Can you work these out from the model? Positions are in its coordinate system, mm. Face numbers are marked on the shaded views. A direction names the side the tool comes from. Give positions to 0.01 mm unless a question says otherwise; leave off trailing zeros. Loops run counter-clockwise (first coordinate to the right, second up) from the corner with the lowest first, then second, coordinate; pieces in that order, holes last. Notation, with made-up numbers: M 74,40.5 L 117,40.5 A22 cw 117,75.5 Z; hole C 75.5,-28 d2. An arc over 180 degrees is marked long. Use CSV: the item, a comma, the result in double quotes.
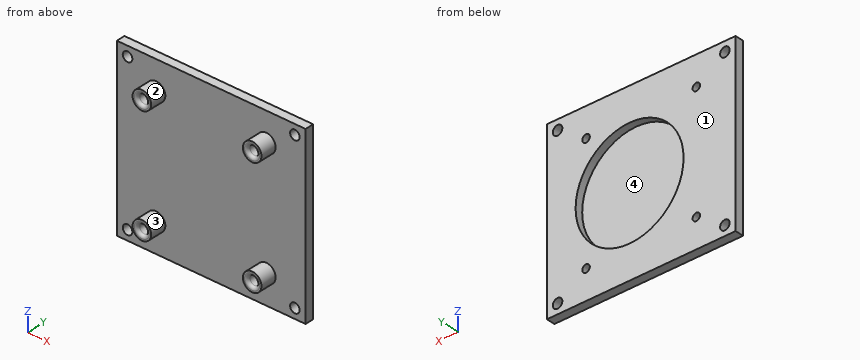
from build123d import *

# Parameters (mm, degrees)
SKETCH3_W           = 65
SKETCH3_H           = 60
BOSS_EXTRUDE3_DEPTH = 3
CUT_EXTRUDE1_REACH  = 57.839
SKETCH4_R           = 1.3
SKETCH9_R           = 3.2
SKETCH9_R_2         = 1.6
BOSS_EXTRUDE5_DEPTH = 5.6
SKETCH10_R          = 18.6
CUT_EXTRUDE3_DEPTH  = 2.6
SKETCH11_R          = 1.65
CUT_EXTRUDE4_DEPTH  = 57.41772771
FILLET1_R           = 1


with BuildPart() as part:
    # Sketch3 → Boss-Extrude3 (new body)
    with BuildSketch(Plane(origin=(0, 0, 0), x_dir=(1, 0, 0), z_dir=(0, 1, 0))):
        with Locations((-14.5, 0)):
            Rectangle(SKETCH3_W, SKETCH3_H)
    extrude(amount=BOSS_EXTRUDE3_DEPTH)

    # Sketch4 → Cut-Extrude1 (cut, up to next)
    with BuildSketch(Plane(origin=(0, 3, 0), x_dir=(1, 0, 0), z_dir=(0, 1, 0)), mode=Mode.PRIVATE) as cut_extrude1_sk1:
        with Locations(Location((-33.5, 20, 0), (0, 0, 270))):
            Circle(SKETCH4_R)
    cut_extrude1_tool1 = extrude(cut_extrude1_sk1.sketch, amount=-CUT_EXTRUDE1_REACH, mode=Mode.PRIVATE) & part.part
    # Sketch4 → Cut-Extrude1 (cut, up to next)
    with BuildSketch(Plane(origin=(0, 3, 0), x_dir=(1, 0, 0), z_dir=(0, 1, 0)), mode=Mode.PRIVATE) as cut_extrude1_sk2:
        with Locations(Location((4.5, 20, 0), (0, 0, 270))):
            Circle(SKETCH4_R)
    cut_extrude1_tool2 = extrude(cut_extrude1_sk2.sketch, amount=-CUT_EXTRUDE1_REACH, mode=Mode.PRIVATE) & part.part
    # Sketch4 → Cut-Extrude1 (cut, up to next)
    with BuildSketch(Plane(origin=(0, 3, 0), x_dir=(1, 0, 0), z_dir=(0, 1, 0)), mode=Mode.PRIVATE) as cut_extrude1_sk3:
        with Locations(Location((4.5, -20, 0), (0, 0, 270))):
            Circle(SKETCH4_R)
    cut_extrude1_tool3 = extrude(cut_extrude1_sk3.sketch, amount=-CUT_EXTRUDE1_REACH, mode=Mode.PRIVATE) & part.part
    # Sketch4 → Cut-Extrude1 (cut, up to next)
    with BuildSketch(Plane(origin=(0, 3, 0), x_dir=(1, 0, 0), z_dir=(0, 1, 0)), mode=Mode.PRIVATE) as cut_extrude1_sk4:
        with Locations(Location((-33.5, -20, 0), (0, 0, 270))):
            Circle(SKETCH4_R)
    cut_extrude1_tool4 = extrude(cut_extrude1_sk4.sketch, amount=-CUT_EXTRUDE1_REACH, mode=Mode.PRIVATE) & part.part
    add(cut_extrude1_tool1.solids().sort_by_distance((-33.5, 3, -20))[0], mode=Mode.SUBTRACT)
    add(cut_extrude1_tool2.solids().sort_by_distance((4.5, 3, -20))[0], mode=Mode.SUBTRACT)
    add(cut_extrude1_tool3.solids().sort_by_distance((4.5, 3, 20))[0], mode=Mode.SUBTRACT)
    add(cut_extrude1_tool4.solids().sort_by_distance((-33.5, 3, 20))[0], mode=Mode.SUBTRACT)

    # Sketch9 → Boss-Extrude5 (add)
    # profile 1 of 4: a face of its own
    with BuildSketch(Plane.XZ):
        with Locations(Location((-33.5, 20, 0), (0, 0, 270))):
            Circle(SKETCH9_R)
        with Locations(Location((-33.5, 20, 0), (0, 0, 270))):
            Circle(SKETCH9_R_2, mode=Mode.SUBTRACT)
    # profile 2 of 4: a face of its own
    with BuildSketch(Plane.XZ):
        with Locations(Location((-33.5, -20, 0), (0, 0, 270))):
            Circle(SKETCH9_R)
        with Locations(Location((-33.5, -20, 0), (0, 0, 270))):
            Circle(SKETCH9_R_2, mode=Mode.SUBTRACT)
    # profile 3 of 4: a face of its own
    with BuildSketch(Plane.XZ):
        with Locations(Location((4.5, 20, 0), (0, 0, 270))):
            Circle(SKETCH9_R)
        with Locations(Location((4.5, 20, 0), (0, 0, 270))):
            Circle(SKETCH9_R_2, mode=Mode.SUBTRACT)
    # profile 4 of 4: a face of its own
    with BuildSketch(Plane.XZ):
        with Locations(Location((4.5, -20, 0), (0, 0, 270))):
            Circle(SKETCH9_R)
        with Locations(Location((4.5, -20, 0), (0, 0, 270))):
            Circle(SKETCH9_R_2, mode=Mode.SUBTRACT)
    extrude(amount=BOSS_EXTRUDE5_DEPTH)

    # Sketch10 → Cut-Extrude3 (cut)
    with BuildSketch(Plane(origin=(0, 3, 0), x_dir=(1, 0, 0), z_dir=(0, 1, 0))):
        with Locations(Location((-10.5, 0, 0), (0, 0, 270))):
            Circle(SKETCH10_R)
    extrude(amount=-CUT_EXTRUDE3_DEPTH, mode=Mode.SUBTRACT)

    # Sketch11 → Cut-Extrude4 (cut, through all)
    with BuildSketch(Plane(origin=(0, 3, 0), x_dir=(1, 0, 0), z_dir=(0, 1, 0))):
        with Locations(Location((14.325982777, -26.608599486, 0), (0, 0, 270))):
            Circle(SKETCH11_R)
        with Locations(Location((-43.325982777, -26.608599486, 0), (0, 0, 270))):
            Circle(SKETCH11_R)
        with Locations(Location((14.325982777, 26.608599486, 0), (0, 0, 270))):
            Circle(SKETCH11_R)
        with Locations(Location((-43.325982777, 26.608599486, 0), (0, 0, 270))):
            Circle(SKETCH11_R)
    extrude(amount=-CUT_EXTRUDE4_DEPTH, mode=Mode.SUBTRACT)

    # Fillet1
    fillet1_edges = [part.edges().sort_by_distance(p)[0] for p in [
        (-33.5, -5.6, 21.6),
        (-33.5, -5.6, -18.4),
        (4.5, -5.6, 21.6),
        (4.5, -5.6, -18.4),
    ]]
    fillet(fillet1_edges, radius=FILLET1_R)


solid = part.part
Q1. If we mould it in two halves opening along X, with no side actions, what happens to the marked faces 1 and 2? For each: released by +X, released by -X, zero draft, split by the parting line, or undercut.
Model answer:
face 1,"zero draft"
face 2,"undercut"
Q2. For the marked faces 3 and 4, which set-ups out of +Z, -Z, +X, -X, +Y, -Y let a thin tool reach every point of the face, with its end or its side?
Model answer:
face 3,"-Y"
face 4,"+Y"
Q3. I want a section at D-D, the plane x = -10.5. Please give me the cut outline in (y, z).
Model answer:
outline,"M 0,-30 L 3,-30 L 3,-18.6 L 0.4,-18.6 L 0.4,18.6 L 3,18.6 L 3,30 L 0,30 Z"
Q4. I want a section at B-B, the plane z = -20. State how many separate pieces and enclosed holes the cut face has, then the cut area to 3 significant figures.
Model answer:
separate pieces,"3"
enclosed holes,"0"
area,"214 mm2"
Q5. I'm going to push flat-ended pins straight in: P1, Ø5, axis at x = 4.5, z = 20, coming from the -Y side (3 decimals); P2, Ø18.5, axis at x = -17.5, z = -3.5, coming from the +Y side; P3, Ø2, axis at x = -43.33, z = 26.61, coming from the +Y side; P4, Ø2, axis at x = 7.5, y = -1.5, coming from the -Z side. Where does each tip first touch, or does it pass through?
Model answer:
P1,"y = -5.595"
P2,"y = 0.4"
P3,"through"
P4,"z = -22.5"
Q6. Please list where these lines run through material, in increasing order: L1, parallel to X at y = 1.6, z = 20; L2, parallel to X at y = 1.5, z = -26.5; L3, parallel to X at y = -2.45, z = 20. Write a range as from..to.
Model answer:
L1,"-47..-34.8, -32.2..3.2, 5.8..18"
L2,"-47..-44.97, -41.68..12.68, 15.97..18"
L3,"-36.7..-35.1, -31.9..-30.3, 1.3..2.9, 6.1..7.7"
Q7. I want a section at A-A, the plane y = -1. Please give me the cut outline in (x, z).
Model answer:
outline,"C -33.5,-20 d6.4; C -33.5,20 d6.4; C 4.5,-20 d6.4; C 4.5,20 d6.4; hole C -33.5,-20 d3.2; hole C -33.5,20 d3.2; hole C 4.5,-20 d3.2; hole C 4.5,20 d3.2"
